Build history of the part. All positions in model axes, mm. A direction names the side the tool comes from. Give positions to 0.01 mm unless a question says otherwise; leave off trailing zeros. Order: outer loops, then holes, each group sorted by start corner. A loop starts at its lowest first (then second) coordinate and runs counter-clockwise, first axis right, second up. Notation, with made-up numbers: (73.25, -35) - (121.25, -35) arc R25 ccw to (121.25, -6) - close; hole circle Ø3 at (16.5, 49.5). An arc over 180 degrees is marked (long way). Use a Markdown table: item, result. Add a question column.
(1) Slice it at C-C (x = 5). Write the cut outline in (y, z), then the cut area to 3 significant figures.
(2) Which spindle directions (+Z, -Z, +X, -X, +Y, -Y) get a long thin tool onto all of the face, cutting with end or side? Do faces 1 (the face through (7.63, -1.86, 3.45)), 2 (the face through (-1.3, -1.3, 4.5)), 3 (the face through (-10.332, -2.075, 3.451)), 4 (the face through (-3.837, 9.815, 3.451)). Say none if no direction does.
(3) Slice it at B-B (y = 9). Write the cut outline in (x, z).
(4) Flat gauge pins, fed straight in: pin 1 (5 mm diameter, centred on x = 0, y = 0, fed in from -Z); pin 2 (3 mm diameter, centred on y = 3, z = 3, fed in from +X); pin 3 (2 mm diameter, centred on y = -9, z = 6, fed in from +X). Where does each tip first touch, or does it go through?
(5) Wall check: line 1 (X direction, y = 0.5, z = 1.25); line 2 (X direction, y = 0.25, z = 6.5); line 3 (Y direction, x = 1.75, z = 0.5). Give the ranges that are in metal, low to high.
(6) Mould opens along X. For faces 5 (the face through (10.418, -1.584, 3.451)), 6 (the face through (3, 2, 0)), 7 (the face through (8.999, 5.483, 3.451)), 8 (the face through (-6.868, -3.854, 3.451)) say: +X half, -X half, draft (parallel to the pull), parting line (faces both ways), or undercut.
(7) Slice it at A-A (y = -9.25). Write the cut outline in (x, z).
from build123d import *

# Parameters (mm, degrees)
CROQUIS1_R              = 12
CROQUIS1_R_2            = 10
CROQUIS1_R_3            = 3
CROQUIS1_R_4            = 1.5
SALIENTE_EXTRUIR1_DEPTH = 7
CORTAR_EXTRUIR2_DEPTH   = 7
MATRIZC2_COUNT          = 9
CROQUIS3_R              = 1.5
CORTAR_EXTRUIR3_DEPTH   = 7
CROQUIS7_R              = 3
CORTAR_EXTRUIR4_DEPTH   = 4.5


with BuildPart() as part:
    # Croquis1 → Saliente-Extruir1 (new body)
    # profile 1 of 4: a face of its own
    with BuildSketch(Plane(origin=(0, 0, 0), x_dir=(0, 1, 0), z_dir=(0, 0, 1))):
        with Locations(Location((0, 0, 0), (0, 0, 90))):
            Circle(CROQUIS1_R)
        Circle(CROQUIS1_R_2, mode=Mode.SUBTRACT)
    # profile 2 of 4: a face of its own
    with BuildSketch(Plane(origin=(0, 0, 0), x_dir=(0, 1, 0), z_dir=(0, 0, 1))):
        Circle(CROQUIS1_R_2)
        Circle(CROQUIS1_R_3, mode=Mode.SUBTRACT)
    # profile 3 of 4: a face of its own
    with BuildSketch(Plane(origin=(0, 0, 0), x_dir=(0, 1, 0), z_dir=(0, 0, 1))):
        Circle(CROQUIS1_R_3)
        Circle(CROQUIS1_R_4, mode=Mode.SUBTRACT)
    # profile 4 of 4: a face of its own
    with BuildSketch(Plane(origin=(0, 0, 0), x_dir=(0, 1, 0), z_dir=(0, 0, 1))):
        Circle(CROQUIS1_R_4)
    extrude(amount=SALIENTE_EXTRUIR1_DEPTH)

    # Croquis2 → Cortar-Extruir2 (cut)
    with BuildSketch(Plane(origin=(0, 0, 0), x_dir=(-1, 0, 0), z_dir=(0, 0, -1))):
        with BuildLine():
            ThreePointArc((-1.671726175, -11.882984961), (2.52, -11.732416631), (6.40384449, -10.148437108))
            ThreePointArc((6.40384449, -10.148437108), (4.588589795, -9.529007631), (3.392213046, -8.029832803))
            ThreePointArc((3.392213046, -8.029832803), (2.772460995, -7.361306204), (1.866050022, -7.264148767))
            ThreePointArc((1.866050022, -7.264148767), (1.575, -7.332760394), (1.281446283, -7.389715517))
            ThreePointArc((1.281446283, -7.389715517), (0.494876961, -7.850507358), (0.204307181, -8.714561536))
            ThreePointArc((0.204307181, -8.714561536), (-0.270936109, -10.57278281), (-1.671726175, -11.882984961))
        make_face()
    cortar_extruir2 = extrude(amount=-CORTAR_EXTRUIR2_DEPTH, mode=Mode.SUBTRACT)

    # MatrizC2: Cortar-Extruir2 ×9 about axis
    matrizc2_axis = Axis((0, 0, 0), (0, 0, 1))
    for i in range(1, MATRIZC2_COUNT):
        add(cortar_extruir2.rotate(matrizc2_axis, i * 360 / MATRIZC2_COUNT), mode=Mode.SUBTRACT)

    # Croquis3 → Cortar-Extruir3 (cut)
    with BuildSketch(Plane(origin=(0, 0, 0), x_dir=(-1, 0, 0), z_dir=(0, 0, -1))):
        Circle(CROQUIS3_R)
    extrude(amount=-CORTAR_EXTRUIR3_DEPTH, mode=Mode.SUBTRACT)

    # Croquis7 → Cortar-Extruir4 (cut)
    with BuildSketch(Plane(origin=(0, 0, 0), x_dir=(-1, 0, 0), z_dir=(0, 0, -1))):
        Circle(CROQUIS7_R)
    extrude(amount=-CORTAR_EXTRUIR4_DEPTH, mode=Mode.SUBTRACT)


solid = part.part
Solution:
| question | item | result |
|---|---|---|
| 1 | outline | (-6.44, 0) - (5.96, 0) - (5.96, 7) - (-6.44, 7) - close |
| 1 | area | 86.8 mm2 |
| 2 | face 1 | +Z, -Z |
| 2 | face 2 | -Z |
| 2 | face 3 | +Z, -Z, -X |
| 2 | face 4 | +Z, -Z, +Y |
| 3 | outline | (-5.97, 0) - (-3.13, 0) - (-3.13, 7) - (-5.97, 7) - close; (0.47, 0) - (3.4, 0) - (3.4, 7) - (0.47, 7) - close |
| 4 | pin 1 | z = 4.5 |
| 4 | pin 2 | x = 8.14 |
| 4 | pin 3 | x = 8.89 |
| 5 | line 1 | -7.48 to -2.96, 2.96 to 11.05 |
| 5 | line 2 | -7.5 to -1.48, 1.48 to 11.37 |
| 5 | line 3 | -11.76 to -2.44, 2.44 to 11.26 |
| 6 | face 5 | undercut |
| 6 | face 6 | draft |
| 6 | face 7 | +X half |
| 6 | face 8 | undercut |
| 7 | outline | (-6.61, 0) - (-4.24, 0) - (-4.24, 7) - (-6.61, 7) - close; (-0.18, 0) - (2.72, 0) - (2.72, 7) - (-0.18, 7) - close |
